Read the model definition and answer for the solid it produces. Units are mm, in the model's axes. Face numbers are marked on the shaded views. A direction names the side the tool comes from. Give positions to 0.01 mm unless a question says otherwise; leave off trailing zeros. Loops run counter-clockwise (first coordinate to the right, second up) from the corner with the lowest first, then second, coordinate; pieces in that order, holes last. Notation, with made-up numbers: (-36, 56) - (-22, 56) arc R15 cw to (-22, 70) - close; hole circle Ø9 at (63.25, 21). An arc over 180 degrees is marked (long way). Write item = value, one per line.
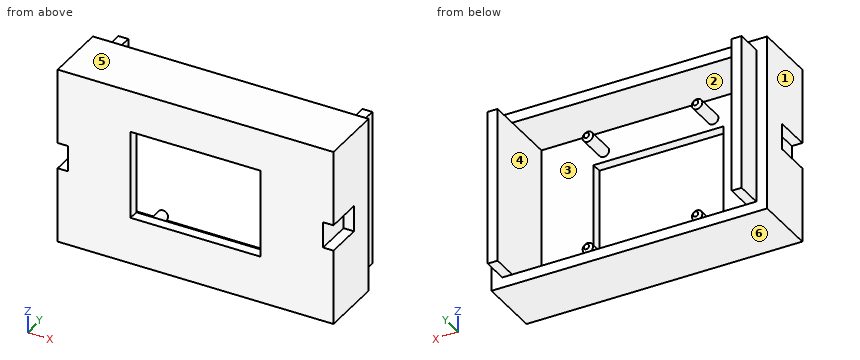
```python
from build123d import *

# Parameters (mm, degrees)
SKETCH_1_W                         = 29
SKETCH_1_H                         = 30
SKETCH_1_W_2                       = 25
SKETCH_1_H_2                       = 17
EXTRUDE_1_DEPTH                    = 2
SKETCH_4_R                         = 1
EXTRUDE_2_DEPTH                    = 6
CHAMFER_1_SIZE                     = 0.5
PATTERN_LINEAR_1_COUNT             = 2
PATTERN_LINEAR_1_PITCH             = 21
PATTERN_LINEAR_1_COUNT_DIR2        = 2
PATTERN_LINEAR_1_PITCH_DIR2        = 22
CHAMFER_1_OF_PATTERN_LINEAR_1_SIZE = 0.5
SKETCH_5_W                         = 53
SKETCH_5_H                         = 34
SKETCH_5_W_2                       = 29
SKETCH_5_H_2                       = 30
EXTRUDE_3_DEPTH                    = 2
SKETCH_6_W                         = 53
SKETCH_6_H                         = 34
SKETCH_6_W_2                       = 45
SKETCH_6_H_2                       = 30
EXTRUDE_4_DEPTH                    = 10
SKETCH_7_W                         = 1.9
SKETCH_7_H                         = 30
EXTRUDE_5_DEPTH                    = 5
SKETCH_8_W                         = 5
SKETCH_8_H                         = 7
CUT_EXTRUDE_1_DEPTH                = 2
CUT_EXTRUDE_2_DEPTH                = 1


with BuildPart() as part:
    # 草图1 → 凸台-拉伸1 (new body)
    with BuildSketch(Plane(origin=(0, 0, 0), x_dir=(1, 0, 0), z_dir=(0, 1, 0))):
        with Locations((14.5, 15)):
            Rectangle(SKETCH_1_W, SKETCH_1_H)
        with Locations((14.5, 14.5)):
            Rectangle(SKETCH_1_W_2, SKETCH_1_H_2, mode=Mode.SUBTRACT)
    extrude(amount=EXTRUDE_1_DEPTH)

    # 草图4 → 凸台-拉伸2 (add)
    with BuildSketch(Plane(origin=(0, 2, 0), x_dir=(1, 0, 0), z_dir=(0, 1, 0))):
        with Locations(Location((4, 26, 0), (0, 0, 90))):
            Circle(SKETCH_4_R)
    extrude_2 = extrude(amount=EXTRUDE_2_DEPTH)

    # 倒角1
    chamfer_1_edges = [part.edges().sort_by_distance(p)[0] for p in [
        (4, 8, -25),
    ]]
    chamfer(chamfer_1_edges, length=CHAMFER_1_SIZE)

    # 阵列(线性)1: Extrude 2 2 × 2
    with Locations(*[(i * PATTERN_LINEAR_1_PITCH, 0, j * PATTERN_LINEAR_1_PITCH_DIR2) for i in range(PATTERN_LINEAR_1_COUNT) for j in range(PATTERN_LINEAR_1_COUNT_DIR2) if (i, j) != (0, 0)]):
        add(extrude_2)

    # 倒角1 of 阵列(线性)1
    chamfer_1_of_pattern_linear_1_edges = [part.edges().sort_by_distance(p)[0] for p in [
        (4, 8, -3),
        (25, 8, -25),
        (25, 8, -3),
    ]]
    chamfer(chamfer_1_of_pattern_linear_1_edges, length=CHAMFER_1_OF_PATTERN_LINEAR_1_SIZE)

    # 草图5 → 凸台-拉伸3 (add)
    with BuildSketch(Plane.XZ):
        with Locations((14.5, -15)):
            Rectangle(SKETCH_5_W, SKETCH_5_H)
        with Locations((14.5, -15)):
            Rectangle(SKETCH_5_W_2, SKETCH_5_H_2, mode=Mode.SUBTRACT)
    extrude(amount=-EXTRUDE_3_DEPTH)

    # 草图6 → 凸台-拉伸4 (add)
    with BuildSketch(Plane(origin=(0, 2, 0), x_dir=(1, 0, 0), z_dir=(0, 1, 0))):
        with Locations((14.5, 15)):
            Rectangle(SKETCH_6_W, SKETCH_6_H)
        with Locations((14.5, 15)):
            Rectangle(SKETCH_6_W_2, SKETCH_6_H_2, mode=Mode.SUBTRACT)
    extrude(amount=EXTRUDE_4_DEPTH)

    # 草图7 → 凸台-拉伸5 (add)
    with BuildSketch(Plane(origin=(0, 12, 0), x_dir=(1, 0, 0), z_dir=(0, 1, 0))):
        with Locations((-8.95, 15)):
            Rectangle(SKETCH_7_W, SKETCH_7_H)
        with Locations((37.95, 15)):
            Rectangle(SKETCH_7_W, SKETCH_7_H)
    extrude(amount=EXTRUDE_5_DEPTH)

    # 草图8 → 切除-拉伸1 (cut)
    with BuildSketch(Plane.ZY.offset(12)):
        with Locations((-15, 3.5)):
            Rectangle(SKETCH_8_W, SKETCH_8_H)
    cut_extrude_1 = extrude(amount=-CUT_EXTRUDE_1_DEPTH, mode=Mode.SUBTRACT)

    # 草图9 → 切除-拉伸2 (cut)
    with BuildSketch(Plane(origin=(0, 2, 0), x_dir=(1, 0, 0), z_dir=(0, 1, 0))):
        with BuildLine():
            Line((14.558917537, 25.486895376), (14.412742382, 25.486895376))
            Line((14.412742382, 25.486895376), (14.412742382, 28.945131046))
            Line((14.412742382, 28.945131046), (14.141274238, 28.708715108))
            add(Edge.make_bspline(
                [(14.141274238, 28.708715108), (14.131226678, 28.699624795), (14.111776808, 28.682027946), (14.078955395, 28.667696389), (14.049596625, 28.660757409), (14.025482894, 28.674909055), (14.024334353, 28.706256057), (14.027312724, 28.742599315), (14.035982745, 28.785479878), (14.049247389, 28.811861074), (14.055508204, 28.824312806)],
                knots=[0, 0, 0, 0, 1.145827462, 2.218070327, 3.049383638, 3.602329049, 4.338402789, 5.486582277, 6.813685142, 8, 8, 8, 8], degree=3))
            Line((14.055508204, 28.824312806), (14.478372043, 29.619326657))
            Line((14.478372043, 29.619326657), (14.911676966, 28.849669721))
            add(Edge.make_bspline(
                [(14.911676966, 28.849669721), (14.920492206, 28.831763899), (14.93731818, 28.7975864), (14.949542857, 28.753205391), (14.955311509, 28.721793647), (14.95568764, 28.70307516), (14.95245501, 28.688159671), (14.942591019, 28.675147665), (14.922248283, 28.667540916), (14.896003584, 28.678587323), (14.868455455, 28.697222198), (14.850537253, 28.714349218), (14.840826763, 28.72363094)],
                knots=[0, 0, 0, 0, 1.968558185, 3.757459298, 4.529049772, 5.118788489, 5.601560465, 6.004578554, 6.689087708, 7.559937433, 8.677646168, 10, 10, 10, 10], degree=3))
            Line((14.840826763, 28.72363094), (14.558917537, 28.960046878))
            Line((14.558917537, 28.960046878), (14.558917537, 25.486895376))
        make_face()
    extrude(amount=-CUT_EXTRUDE_2_DEPTH, mode=Mode.SUBTRACT)

    # 镜向1: 切除-拉伸1 across plane
    add(cut_extrude_1.mirror(Plane.ZY.offset(-14.5)), mode=Mode.SUBTRACT)


solid = part.part
```
1) A cutting plane is placed at C-C on x = 9.5. Determine the outline of the cut face in (y, z).
Output:
outline = (0, -32) - (12, -32) - (12, -30) - (2, -30) - (2, -23) - (0, -23) - close; (0, -6) - (2, -6) - (2, 0) - (12, 0) - (12, 2) - (0, 2) - close
2) The mould has two halves that part along Z. Classify the marked faces 3, 4, 5 and 6: pulls with the +Z half, pulls with the -Z half, needs draft (parallel to the pull), parting line crosses it, or undercut.
Output:
face_3 = undercut
face_4 = undercut
face_5 = pulls with the +Z half
face_6 = pulls with the -Z half
3) A cutting plane is placed at B-B on z = -9. Determine the outline of the cut face in (x, y), then the cut area to 3 significant figures.
Output:
outline = (-12, 0) - (2, 0) - (2, 2) - (-8, 2) - (-8, 17) - (-9.9, 17) - (-9.9, 12) - (-12, 12) - close; (27, 0) - (41, 0) - (41, 12) - (38.9, 12) - (38.9, 17) - (37, 17) - (37, 2) - (27, 2) - close
area = 155 mm²
4) A cutting plane is placed at A-A on y = 3.5. Determine the outline of the cut face in (x, z).
Output:
outline = (-12, -32) - (41, -32) - (41, -17.5) - (39, -17.5) - (39, -12.5) - (41, -12.5) - (41, 2) - (-12, 2) - (-12, -12.5) - (-10, -12.5) - (-10, -17.5) - (-12, -17.5) - close; circle Ø2 at (4, -26); circle Ø2 at (4, -4); circle Ø2 at (25, -26); circle Ø2 at (25, -4); hole (-8, -30) - (37, -30) - (37, 0) - (-8, 0) - close
5) Each of these flat-tipped pins is pushed along its axis until it touches: P1, Ø1.5, axis at y = 3.5, z = -15.5, coming from the -X side; P2, Ø1, axis at y = 15, z = -21.5, coming from the +X side; P3, Ø1.1, axis at x = 4, z = -4, coming from the +Y side. Where does it stop, or does it pass through?
Output:
P1 = -10
P2 = 38.9
P3 = 8
6) Find the intervals of material crossed by probe 1 along X at (y, z) = (1.5, -14.5); probe 2 along Z at (x, y) = (17, 7); probe 3 along X at (y, z) = (1.75, -11), in increasing order.
Output:
probe_1 = -10 to 2, 27 to 39
probe_2 = -32 to -30, 0 to 2
probe_3 = -12 to 2, 27 to 41
7) A cutting plane is placed at D-D on y = 9.5. Determine the outline of the cut face in (x, z), then the cut area to 3 significant figures.
Output:
outline = (-12, -32) - (41, -32) - (41, 2) - (-12, 2) - close; hole (-8, -30) - (37, -30) - (37, 0) - (-8, 0) - close
area = 452 mm²
8) A tool of negligible diameter and unlimited length cuts with its end or side. For the marked faces 1 and 2, from which of +Z, -Z, +X, -X, +Y, -Y can it reach the whole face along a straight path? Write none if from no direction.
Output:
face_1 = +Z, -Z, -X, +Y, -Y
face_2 = +Y
